Input: dimensioned drawing with shaded views. Units: mm. Origin: part minimum x, y, z. A direction names the side the tool comes from. Round coordinates to 2 decimals unless told otherwise and drop trailing zeros. Loops run counter-clockwise (first coordinate to the right, second up) from the corner with the lowest first, then second, coordinate; pieces in that order, holes last. Notation, with made-up numbers: M 77,-3 L 84,-3 A27 ccw 84,22 Z; hole C 22,77.5 d3. An arc over 180 degrees is marked long. Put each result on its own line as item: value. Start each with the question number.
1) Section C-C on x = 23. Output: boundary loops of the cut face in (y, z), plus the area to 3 significant figures.
2) Reachability of the marked faces 4 and 5 from +Z, -Z, +X, -X, +Y, -Y: full face, straight path, thin tool, end or side. Return the list, or none.
3) Draft query along Z for the marked faces 1, 2 and 3. Return one class per face: +Z half, -Z half, draft (parallel to the pull), parting line (faces both ways), or undercut.
4) Line query: probe 1 along Z at (x, y) = (18, 2.9); probe 2 along X at (y, z) = (2.4, 34); probe 3 along Y at (x, z) = (27, 7.5). Output: solid intervals per line, ascending.
5) Section B-B on z = 19. Output: boundary loops of the cut face in (x, y).
6) Section A-A on y = 3.15. Output: boundary loops of the cut face in (x, z).
7) Section D-D on z = 8.5. Output: boundary loops of the cut face in (x, y), plus the area to 3 significant figures.
8) Pin query (flat end, axial travel): pin 1 (1.5 mm diameter, centred on y = 3.5, z = 27, fed in from -X); pin 2 (2 mm diameter, centred on y = 2.5, z = 1.5, fed in from -X); pin 3 (0.9 mm diameter, centred on y = 2.5, z = 30.5, fed in from +X); pin 4 (3 mm diameter, centred on x = 20, z = 9.5, fed in from +Y). Return the tip coordinate at first contact, or that it passes through.
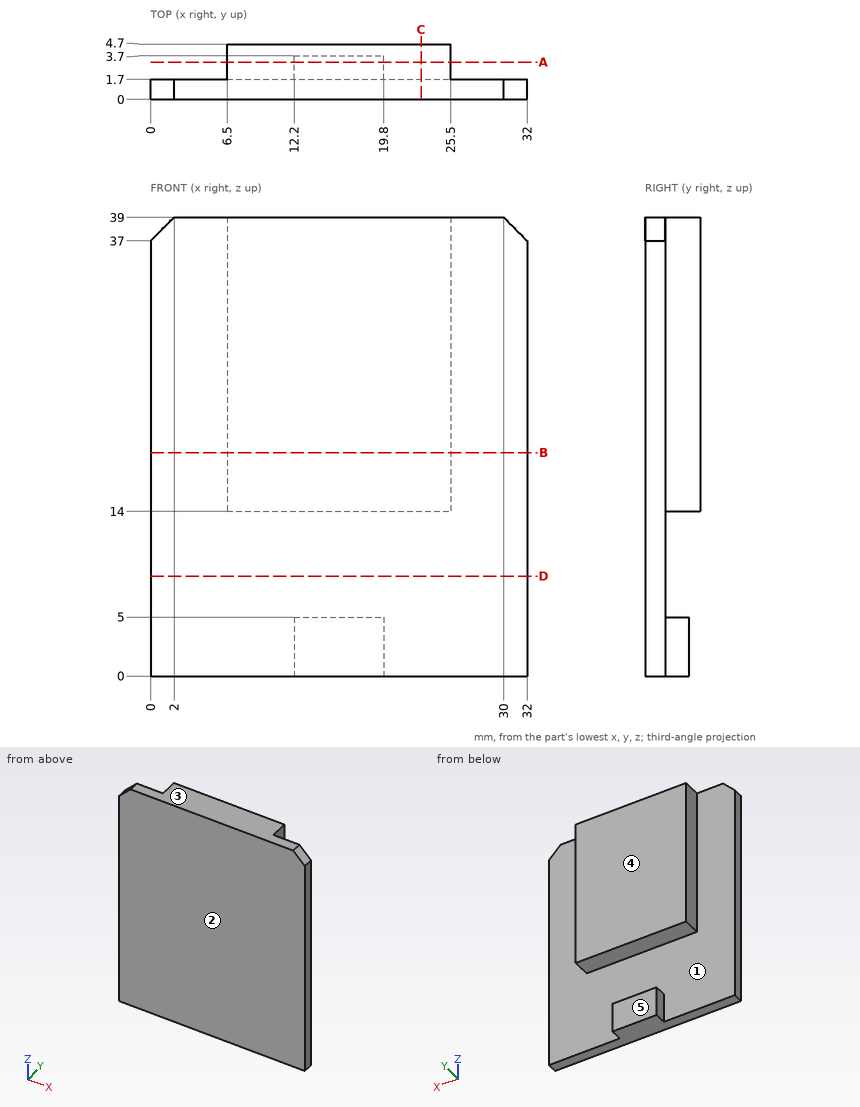
Geometry results:
1. outline: M 0,0 L 1.7,0 L 1.7,14 L 4.7,14 L 4.7,39 L 0,39 Z
1. area: 141 mm²
2. face 4: +Z, -Z, +X, -X, +Y
2. face 5: -Z, +X, -X, +Y
3. face 1: undercut
3. face 2: draft
3. face 3: +Z half
4. probe 1: z = 0 to 5, 14 to 39
4. probe 2: x = 6.5 to 25.5
4. probe 3: y = 0 to 1.7
5. outline: M 0,0 L 32,0 L 32,1.7 L 25.5,1.7 L 25.5,4.7 L 6.5,4.7 L 6.5,1.7 L 0,1.7 Z
6. outline: M 6.5,14 L 25.5,14 L 25.5,39 L 6.5,39 Z; M 12.2,0 L 19.8,0 L 19.8,5 L 12.2,5 Z
7. outline: M 0,0 L 32,0 L 32,1.7 L 0,1.7 Z
7. area: 54.4 mm²
8. pin 1: stops at x = 6.5
8. pin 2: stops at x = 0
8. pin 3: stops at x = 25.5
8. pin 4: stops at y = 1.7
